from build123d import *

# Parameters (mm, degrees)
FILLET_2_R = 0.5
FILLET_3_R = 0.5
FILLET_4_R = 1
FILLET_5_R = 1


with BuildPart() as part:
    # 草图2 → 旋转1 (revolve)
    with BuildSketch(Plane.XY, mode=Mode.PRIVATE) as revolve_1_sk:
        Polygon((-32.84202412, 5), (12.15797588, 5), (12.15797588, 7.5), (12.15797588, 8.732933377), (9.81519701, 8.732933377), (9.36644596, 7.5), (-6.63355404, 7.5), (-8.84202412, 6), (-32.84202412, 6), align=None)
    revolve(revolve_1_sk.sketch.rotate(Axis((-59.135771609, 0, 0), (1, 0, 0)), 90), axis=Axis((-59.135771609, 0, 0), (1, 0, 0)))

    # 圆角2
    fillet_2_edges = [part.edges().sort_by_distance(p)[0] for p in [
        (9.36644596, 0, -7.5),
    ]]
    fillet(fillet_2_edges, radius=FILLET_2_R)

    # 圆角3
    fillet_3_edges = [part.edges().sort_by_distance(p)[0] for p in [
        (9.81519701, 0, -8.732933377),
    ]]
    fillet(fillet_3_edges, radius=FILLET_3_R)

    # 圆角4
    fillet_4_edges = [part.edges().sort_by_distance(p)[0] for p in [
        (-6.63355404, 0, -7.5),
    ]]
    fillet(fillet_4_edges, radius=FILLET_4_R)

    # 圆角5
    fillet_5_edges = [part.edges().sort_by_distance(p)[0] for p in [
        (-8.84202412, 0, -6),
    ]]
    fillet(fillet_5_edges, radius=FILLET_5_R)


solid = part.part
Work out the finished part from the listing and answer in its coordinate system (mm). A direction names the side the tool comes from. Round coordinates to 2 decimals unless told otherwise and drop trailing zeros. Write each loop counter-clockwise with the first axis right and the second up, starting at its lowest first coordinate (ties: lowest second). Pieces come first, ordered by that corner, then holes. Notation, with made-up numbers: M 7.25,-31 L 56.25,-31 A18 ccw 56.25,-15 Z; hole C 58,2.5 d9. An arc over 180 degrees is marked long. Use a Markdown table: item, result.
1) Flat-ended cylindrical pins translate along their axes: pin 1 (1 mm diameter, centred on x = 4, z = -0.5, fed in from +Y); pin 2 (3 mm diameter, centred on x = -9, z = 4.5, fed in from +Y); pin 3 (1.5 mm diameter, centred on y = 1.5, z = -2, fed in from -X); pin 4 (2 mm diameter, centred on x = -23, z = -2.5, fed in from -Y). Find the tip coordinate at first contact, or state that the pin passes through.
Taken from the geometry:
| item | result |
|---|---|
| pin 1 | stops at y = 7.5 |
| pin 2 | stops at y = 5.66 |
| pin 3 | passes through |
| pin 4 | stops at y = -5.81 |
2) The part is cut by section A-A on x = -15. Give the vertices of the cut face in (y, z).
Taken from the geometry:
| item | result |
|---|---|
| outline | C 0,0 d12; hole C 0,0 d10 |
3) The part is cut by section B-B on x = 4. Give the vertices of the cut face in (y, z), plus the area to 3 significant figures.
Taken from the geometry:
| item | result |
|---|---|
| outline | C 0,0 d15; hole C 0,0 d10 |
| area | 98.2 mm2 |
4) Determine the mould class of faces 3 (the face through (-32.842, -4, -4)), 4 (the face through (11.15, -2.62, 8.33)), 5 (the face through (-10, 0, -5)) for opening direction Z: pulls with the +Z half, pulls with the -Z half, needs draft (parallel to the pull), parting line crosses it, or undercut.
Taken from the geometry:
| item | result |
|---|---|
| face 3 | needs draft |
| face 4 | parting line crosses it |
| face 5 | undercut |
5) Which of the six approach directions +Z, -Z, +X, -X, +Y, -Y give full straight-line access (tool end or side, diameter ignored) to faces 1 (the face through (1.238, -2.253, 7.154)), 2 (the face through (12.158, 4, -4))?
Taken from the geometry:
| item | result |
|---|---|
| face 1 | -X |
| face 2 | +Z, -Z, +X, +Y, -Y |
6) Consider line 1 (Y direction, x = -10.5, z = 0.25); line 2 (Y direction, x = -4.5, z = 0); line 3 (Z direction, x = -25, y = 2). Determine where each line is inside the solid, lowest interval first. Write a range as [from, to].
Taken from the geometry:
| item | result |
|---|---|
| line 1 | y = [-5.99, -4.99], [4.99, 5.99] |
| line 2 | y = [-7.5, -5], [5, 7.5] |
| line 3 | z = [-5.66, -4.58], [4.58, 5.66] |
